from build123d import *

# Parameters (mm, degrees)
SKETCH_1_R               = 84.75
SKETCH_1_R_2             = 2
EXTRUDE_1_DEPTH          = 1.4
CUT_EXTRUDE_1_DEPTH      = 1.4
PATTERN_CIRCULAR_1_COUNT = 12


with BuildPart() as part:
    # Эскиз1 → Бобышка-Вытянуть1 (new body)
    with BuildSketch(Plane.XY):
        Circle(SKETCH_1_R)
        with Locations((15, 45)):
            Circle(SKETCH_1_R_2, mode=Mode.SUBTRACT)
        with Locations((-35, 45)):
            Circle(SKETCH_1_R_2, mode=Mode.SUBTRACT)
        with Locations((-35, -45)):
            Circle(SKETCH_1_R_2, mode=Mode.SUBTRACT)
        with Locations((15, -45)):
            Circle(SKETCH_1_R_2, mode=Mode.SUBTRACT)
    extrude(amount=EXTRUDE_1_DEPTH)

    # Эскиз2 → Вырез-Вытянуть1 (cut)
    with BuildSketch(Plane.XY.offset(1.4)):
        with BuildLine():
            Line((73.45, -14.55), (73.45, 14.55))
            ThreePointArc((73.45, 14.55), (75.05, 16.15), (76.65, 14.55))
            Line((76.65, 14.55), (76.65, -14.55))
            ThreePointArc((76.65, -14.55), (75.05, -16.15), (73.45, -14.55))
        make_face()
    cut_extrude_1 = extrude(amount=-CUT_EXTRUDE_1_DEPTH, mode=Mode.SUBTRACT)

    # Круговой массив1: Вырез-Вытянуть1 ×12 about axis
    pattern_circular_1_axis = Axis((0, 0, 0), (0, 0, 1))
    for i in range(1, PATTERN_CIRCULAR_1_COUNT):
        add(cut_extrude_1.rotate(pattern_circular_1_axis, i * 360 / PATTERN_CIRCULAR_1_COUNT), mode=Mode.SUBTRACT)


solid = part.part
Model file for the job. Use its own axes, mm. A direction names the side the tool comes from. Round coordinates to 2 decimals unless told otherwise and drop trailing zeros. Order: outer loops, then holes, each group sorted by start corner. A loop starts at its lowest first (then second) coordinate and runs counter-clockwise, first axis right, second up. Notation, with made-up numbers: M 53.5,-1 L 112.5,-1 A24 ccw 112.5,15 Z; hole C -24,64.25 d9. An arc over 180 degrees is marked long. Write each question's results on one line, items separated by ' | '. Start each with the question number.
(1) Which spindle directions (+Z, -Z, +X, -X, +Y, -Y) get a long thin tool onto all of the face, cutting with end or side? Do faces 3 (the face through (-38.15, -66.48, 0.71)), 4 (the face through (-1, 1, 1.4)). Say none if no direction does.
(2) Drop flat-ended pins along their axis: pin 1 (6.5 mm diameter, centred on x = 15, y = -45, fed in from +Z); pin 2 (0.7 mm diameter, centred on x = -1, z = 0.5, fed in from -Y). Give the stop position or say it passes through.
(3) Saw through at A-A, the plane x = 0. Give the cut face in (y, z).
(4) Saw through at C-C, the plane y = 45. Give the cut face in (x, z), then the cut area to 3 significant figures.
(5) Probe probe 1 along Y at (x, z) = (30.5, 1.35); probe 2 along X at (y, z) = (11.5, 0.15); probe 3 along Y at (x, z) = (-41, 0.65). List the from-to ranges inside material, lowest first. Write a range as from..to.
(6) Two-plate mould, pull along Y, no slides. Class faces 1 (the face through (63.51, -36.9, 0.71)), 2 (the face through (-1, 1, 0)): pulls with the +Y half, pulls with the -Y half, needs draft (parallel to the pull), parting line crosses it, or undercut.
(7) Saw through at D-D, the plane z = 0.75. State how many separate pieces and enclosed holes the cut face has, then the cut area to 3 significant figures.
Established:
1) face 3: +Z, -Z | face 4: +Z, +X, -X, +Y, -Y
2) pin 1: stops at z = 1.4 | pin 2: stops at y = -84.75
3) outline: M -84.75,0 L -76.65,0 L -76.65,1.4 L -84.75,1.4 Z; M -73.45,0 L 73.45,0 L 73.45,1.4 L -73.45,1.4 Z; M 76.65,0 L 84.75,0 L 84.75,1.4 L 76.65,1.4 Z
4) outline: M -71.82,0 L -62.53,0 L -62.53,1.4 L -71.82,1.4 Z; M -58.83,0 L -37,0 L -37,1.4 L -58.83,1.4 Z; M -33,0 L 13,0 L 13,1.4 L -33,1.4 Z; M 17,0 L 58.83,0 L 58.83,1.4 L 17,1.4 Z; M 62.53,0 L 71.82,0 L 71.82,1.4 L 62.53,1.4 Z | area: 180 mm^2
5) probe 1: y = -79.07..-70.9, -67.2..67.2, 70.9..79.07 | probe 2: x = -83.97..-76.65, -73.45..73.45, 76.65..83.97 | probe 3: y = -74.17..-64.84, -61.14..61.14, 64.84..74.17
6) face 1: undercut | face 2: needs draft
7) separate pieces: 1 | enclosed holes: 16 | area: 21,300 mm^2
